```python
from build123d import *

# Parameters (mm, degrees)
SKETCH1_W           = 76.2
SKETCH1_H           = 12.7
BOSS_EXTRUDE1_DEPTH = 25.4
FILLET1_R           = 5.08


with BuildPart() as part:
    # Sketch1 → Boss-Extrude1 (new body)
    with BuildSketch(Plane.XY):
        Polygon((44.45, 12.7), (13.6906, 12.7), (99.855246, 78.474538932), (95.983665425, 83.546309485), (3.175, 12.7), (3.175, 83.82), (-3.175, 83.82), (-3.175, 12.7), (-95.983665425, 83.546309485), (-99.855246, 78.474538932), (-13.6906, 12.7), (-44.45, 12.7), (-44.45, 3.175), (-101.6, 3.175), (-101.6, -3.175), (-44.45, -3.175), (-44.45, -12.7), (-13.6906, -12.7), (-99.855246, -78.474538932), (-95.983665425, -83.546309485), (-3.175, -12.7), (-3.175, -83.82), (3.175, -83.82), (3.175, -12.7), (95.983665425, -83.546309485), (99.855246, -78.474538932), (13.6906, -12.7), (44.45, -12.7), (44.45, -3.175), (101.6, -3.175), (101.6, 3.175), (44.45, 3.175), align=None)
        Rectangle(SKETCH1_W, SKETCH1_H, mode=Mode.SUBTRACT)
    extrude(amount=BOSS_EXTRUDE1_DEPTH)

    # Fillet1
    fillet1_edges = [part.edges().sort_by_distance(p)[0] for p in [
        (44.45, 12.7, 12.7),
        (44.45, -12.7, 12.7),
        (-44.45, -12.7, 12.7),
        (-44.45, 12.7, 12.7),
    ]]
    fillet(fillet1_edges, radius=FILLET1_R)


solid = part.part
```
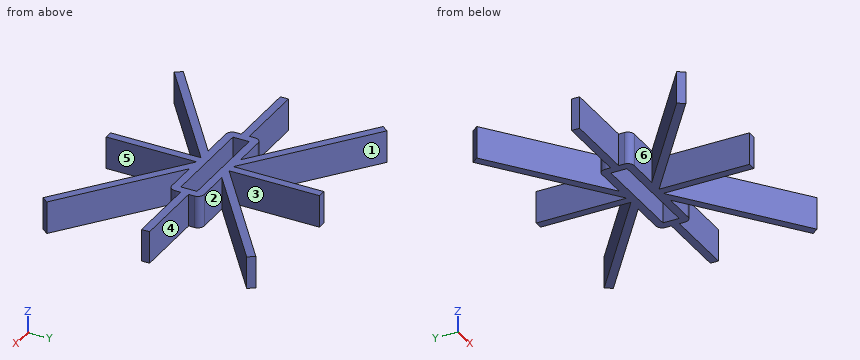
Model file for the job. Use its own axes, mm. Face numbers are marked on the shaded views. A direction names the side the tool comes from. Round coordinates to 2 decimals unless told otherwise and drop trailing zeros. Order: outer loops, then holes, each group sorted by start corner. A loop starts at its lowest first (then second) coordinate and runs counter-clockwise, first axis right, second up. Notation, with made-up numbers: (-23, -27) -> (33, -27) arc R24 cw to (33, 5) -> close; hole circle Ø3 at (14.25, 64). An arc over 180 degrees is marked (long way). Use one line per item in the form item = value.
Item 1: Flat gauge pins, fed straight in: pin 1 Ø2 at (y, z) = (4.5, 14.5) entering from +X; pin 2 Ø12.5 at (x, z) = (61, 10.5) entering from -Y; pin 3 Ø12 at (x, z) = (63.5, 17.5) entering from +Y; pin 4 Ø10 at (x, y) = (50.5, 17) entering from -Z. Where does each tip first touch, or does it go through?
Returned:
pin_1 = 44.45
pin_2 = -61.61
pin_3 = 63.33
pin_4 = through
Item 2: Cut at A-A, the plane x = 11. Write the cut outline in (y, z).
Returned:
outline = (-18.67, 0) -> (-6.35, 0) -> (-6.35, 25.4) -> (-18.67, 25.4) -> close; (6.35, 0) -> (18.67, 0) -> (18.67, 25.4) -> (6.35, 25.4) -> close
Item 3: Tool access for the marked faces 4, 5 and 6: list every direction of +Z, -Z, +X, -X, +Y, -Y with a clear straight run to the whole face (end or side of a thin tool).
Returned:
face_4 = +Z, -Z, +X
face_5 = +Z, -Z, -Y
face_6 = +Z, -Z, -X
Item 4: Cut at C-C, the plane x = 64. Write the cut outline in (y, z) (3 decimals), and give its area (3 significant figures).
Returned:
outline = (-59.131, 0) -> (-51.104, 0) -> (-51.104, 25.4) -> (-59.131, 25.4) -> close; (-3.175, 0) -> (3.175, 0) -> (3.175, 25.4) -> (-3.175, 25.4) -> close; (51.104, 0) -> (59.131, 0) -> (59.131, 25.4) -> (51.104, 25.4) -> close
area = 569 mm^2
Item 5: Pull direction Y, two halves, no side cores. Call the marked faces 1, 2 and 3: released by +Y, released by -Y, zero draft, split by the parting line, or undercut.
Returned:
face_1 = released by +Y
face_2 = undercut
face_3 = zero draft
Item 6: Drill centre lines: line 1 (Y direction, x = -1, z = 21); line 2 (X direction, y = 50.5, z = 22.5) (3 decimals); line 3 (Y direction, x = 76, z = 11.75) (3 decimals). Where is each one in solid material? Low to high.
Returned:
line_1 = -83.82 to -6.35, 6.35 to 83.82
line_2 = -63.209 to -52.693, -3.175 to 3.175, 52.693 to 63.209
line_3 = -68.292 to -60.264, -3.175 to 3.175, 60.264 to 68.292
Item 7: Cut at B-B, the plane y = 43.5. Write the cut outline in (x, z) (3 decimals).
Returned:
outline = (-54.039, 0) -> (-43.523, 0) -> (-43.523, 25.4) -> (-54.039, 25.4) -> close; (-3.175, 0) -> (3.175, 0) -> (3.175, 25.4) -> (-3.175, 25.4) -> close; (43.523, 0) -> (54.039, 0) -> (54.039, 25.4) -> (43.523, 25.4) -> close
